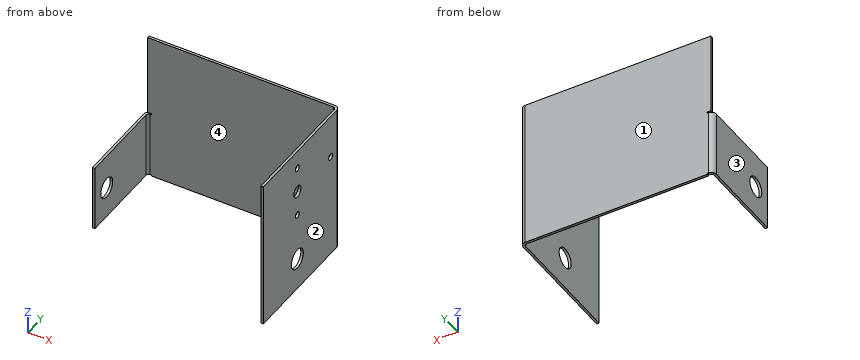
from build123d import *

# Parameters (mm, degrees)
SKETCH1_W                     = 75
SKETCH1_H                     = 60
BASE_FLANGE1_DEPTH            = 1
EDGE_FLANGE1_STRIP_W          = 6
EDGE_FLANGE1_STRIP_H          = 1
EDGE_FLANGE1_STRIP_CUT_DEPTH  = 60
EDGE_FLANGE1_DEPTH            = 60
EDGE_FLANGE3_STRIP_W          = 6
EDGE_FLANGE3_STRIP_H          = 1
EDGE_FLANGE3_STRIP_CUT_DEPTH  = 26.369340124
EDGE_FLANGE3_RELIEF_W         = 6.5
EDGE_FLANGE3_RELIEF_H         = 0.5
EDGE_FLANGE3_RELIEF_CUT_DEPTH = 1
EDGE_FLANGE3_DEPTH            = 26.369340124
SKETCH15_R                    = 1.27
SKETCH15_R_2                  = 2.3749
SKETCH15_R_3                  = 3.975
CUT_EXTRUDE4_DEPTH            = 98.10818709


# Sheet-metal steps are written as plain solids
with BuildPart() as part:
    # Sketch1 → Base-Flange1 (new body)
    with BuildSketch(Plane(origin=(0, 0, 0), x_dir=(1, 0, 0), z_dir=(0, 1, 0))):
        Rectangle(SKETCH1_W, SKETCH1_H)
    extrude(amount=-BASE_FLANGE1_DEPTH)

    # Edge-Flange1 strip (across the edge) → Edge-Flange1 strip cut (cut)
    with BuildSketch(Plane(origin=(37.5, -1, -30), x_dir=(-1, 0, 0), z_dir=(0, 0, 1))):
        with Locations((-2, -0.5)):
            Rectangle(EDGE_FLANGE1_STRIP_W, EDGE_FLANGE1_STRIP_H)
    extrude(amount=EDGE_FLANGE1_STRIP_CUT_DEPTH, mode=Mode.SUBTRACT)

    # Edge-Flange1 section (across the edge) → Edge-Flange1 (add)
    with BuildSketch(Plane(origin=(37.5, -1, -30), x_dir=(-1, 0, 0), z_dir=(0, 0, 1))):
        with BuildLine():
            Line((-1, 1), (-1, 50))
            Line((-1, 50), (0, 50))
            Line((0, 50), (0, 1))
            ThreePointArc((0, 1), (0.292893219, 0.292893219), (1, 0))
            Line((1, 0), (1, -1))
            ThreePointArc((1, -1), (-0.414213562, -0.414213562), (-1, 1))
        make_face()
    extrude(amount=EDGE_FLANGE1_DEPTH)

    # Edge-Flange3 strip (across the edge) → Edge-Flange3 strip cut (cut)
    with BuildSketch(Plane(origin=(-37.5, -1, -3.224868286), x_dir=(1, 0, 0), z_dir=(0, 0, -1))):
        with Locations((-2, -0.5)):
            Rectangle(EDGE_FLANGE3_STRIP_W, EDGE_FLANGE3_STRIP_H)
    extrude(amount=EDGE_FLANGE3_STRIP_CUT_DEPTH, mode=Mode.SUBTRACT)

    # Edge-Flange3 relief (on the sheet) → Edge-Flange3 relief cut (cut)
    with BuildSketch(Plane(origin=(-36.5, -1, -3.224868286), x_dir=(1, 0, 0), z_dir=(0, -1, 0))):
        with Locations((-2.75, 0.25)):
            Rectangle(EDGE_FLANGE3_RELIEF_W, EDGE_FLANGE3_RELIEF_H)
        with Locations((-2.75, -26.619340124)):
            Rectangle(EDGE_FLANGE3_RELIEF_W, EDGE_FLANGE3_RELIEF_H)
    extrude(amount=-EDGE_FLANGE3_RELIEF_CUT_DEPTH, mode=Mode.SUBTRACT)

    # Edge-Flange3 section (across the edge) → Edge-Flange3 (add)
    with BuildSketch(Plane(origin=(-37.5, -1, -3.224868286), x_dir=(1, 0, 0), z_dir=(0, 0, -1))):
        with BuildLine():
            Line((-1, 1), (-1, 35.1591326))
            Line((-1, 35.1591326), (0, 35.1591326))
            Line((0, 35.1591326), (0, 1))
            ThreePointArc((0, 1), (0.292893219, 0.292893219), (1, 0))
            Line((1, 0), (1, -1))
            ThreePointArc((1, -1), (-0.414213562, -0.414213562), (-1, 1))
        make_face()
    extrude(amount=EDGE_FLANGE3_DEPTH)

    # Sketch15 → Cut-Extrude4 (cut, through all)
    with BuildSketch(Plane(origin=(38.5, 0, 0), x_dir=(0, 0, -1), z_dir=(1, 0, 0))):
        with Locations(Location((-22.64162, -28.28773, 0), (0, 0, 90))):
            Circle(SKETCH15_R)
        with Locations(Location((-12.43082, -28.28773, 0), (0, 0, 90))):
            Circle(SKETCH15_R_2)
        with Locations(Location((-2.22002, -28.28773, 0), (0, 0, 90))):
            Circle(SKETCH15_R)
        with Locations(Location((-12.43082, -6.11353, 0), (0, 0, 90))):
            Circle(SKETCH15_R)
        with Locations(Location((17.06918, -28.28773, 0), (0, 0, 90))):
            Circle(SKETCH15_R_3)
    extrude(amount=-CUT_EXTRUDE4_DEPTH, mode=Mode.SUBTRACT)


solid = part.part
Build history of the part. All positions in model axes, mm. Face numbers are marked on the shaded views. Round coordinates to 2 decimals unless told otherwise and drop trailing zeros. Write each loop counter-clockwise with the first axis right and the second up, starting at its lowest first coordinate (ties: lowest second). Pieces come first, ordered by that corner, then holes. Notation, with made-up numbers: (4, 8) -> (9, 8) arc R15 ccw to (9, 35) -> close; hole circle Ø7 at (70, -2.5). An arc over 180 degrees is marked (long way). Write item = value, one per line.
(1) Band-saw the part on D-D (x = 19.5). Give the cut face in (y, z), then the cut area to 3 significant figures.
Answer:
outline = (-1, -30) -> (0, -30) -> (0, 30) -> (-1, 30) -> close
area = 60.0 mm2
(2) Band-saw the part on B-B (z = -7). Give the cut face in (x, y).
Answer:
outline = (-38.5, -36.16) -> (-37.5, -36.16) -> (-37.5, -2) arc R1 cw to (-36.5, -1) -> (36.5, -1) arc R1 cw to (37.5, -2) -> (37.5, -51) -> (38.5, -51) -> (38.5, -2) arc R2 ccw to (36.5, 0) -> (-36.5, 0) arc R2 ccw to (-38.5, -2) -> close
(3) Flat gauge pins, fed straight in: pin 1 (0.8 mm diameter, centred on x = -37, y = -0.5, fed in from -Z); pin 2 (8 mm diameter, centred on y = -42, z = 12.5, fed in from -X); pin 3 (1.1 mm diameter, centred on x = -38, z = -11.5, fed in from -Y). Where does each tip first touch, or does it go through?
Answer:
pin_1 = -29.59
pin_2 = 37.5
pin_3 = -36.16
(4) Band-saw the part on C-C (z = -14.5). Give the cut face in (x, y), then the cut area to 3 significant figures.
Answer:
outline = (-38.5, -36.16) -> (-37.5, -36.16) -> (-37.5, -31.32) -> (-38.5, -31.32) -> close; (-38.5, -25.25) -> (-37.5, -25.25) -> (-37.5, -2) arc R1 cw to (-36.5, -1) -> (36.5, -1) arc R1 cw to (37.5, -2) -> (37.5, -25.25) -> (38.5, -25.25) -> (38.5, -2) arc R2 ccw to (36.5, 0) -> (-36.5, 0) arc R2 ccw to (-38.5, -2) -> close; (37.5, -51) -> (38.5, -51) -> (38.5, -31.32) -> (37.5, -31.32) -> close
area = 149 mm2
(5) Probe L1, parallel to X at y = -20, z = -4.5; L2, parallel to X at y = -22, z = 5; L3, parallel to Y at x = 20.5, z = 20. List the from-to ranges inside material, lowest first.
Answer:
L1 = -38.5 to -37.5, 37.5 to 38.5
L2 = 37.5 to 38.5
L3 = -1 to 0
(6) Two-plate mould, pull along X, no slides. Class the marked faces 1, 2, 3 and 4: pulls with the +X half, pulls with the -X half, needs draft (parallel to the pull), parting line crosses it, or undercut.
Answer:
face_1 = needs draft
face_2 = pulls with the +X half
face_3 = pulls with the -X half
face_4 = undercut
(7) Band-saw the part on A-A (y = -21.5). Give the cut face in (x, z).
Answer:
outline = (-38.5, -29.59) -> (-37.5, -29.59) -> (-37.5, -3.22) -> (-38.5, -3.22) -> close; (37.5, -30) -> (38.5, -30) -> (38.5, 30) -> (37.5, 30) -> close
